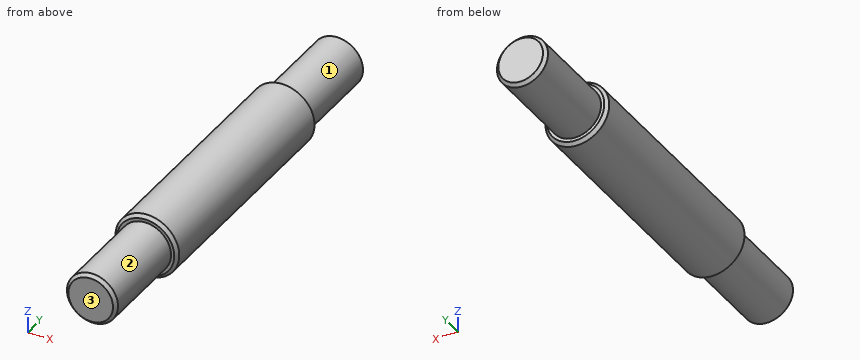
```python
from build123d import *

# Parameters (mm, degrees)
SKETCH1_R           = 5
BOSS_EXTRUDE1_DEPTH = 19
SKETCH2_R           = 4
BOSS_EXTRUDE2_DEPTH = 15
BOSS_EXTRUDE3_START = -53
SKETCH2_2_R         = 4
BOSS_EXTRUDE3_DEPTH = 15
CHAMFER1_SIZE       = 0.5
CHAMFER2_SIZE       = 0.5


with BuildPart() as part:
    # Sketch1 → Boss-Extrude1 (new, symmetric)
    with BuildSketch(Plane(origin=(0, 0, 0), x_dir=(1, 0, 0), z_dir=(0, 1, 0))):
        with Locations(Location((0, 0, 0), (0, 0, 270))):
            Circle(SKETCH1_R)
    extrude(amount=BOSS_EXTRUDE1_DEPTH, both=True)

    # Sketch2 → Boss-Extrude2 (add)
    with BuildSketch(Plane(origin=(0, 19, 0), x_dir=(1, 0, 0), z_dir=(0, 1, 0))):
        with Locations(Location((0, 0, 0), (0, 0, 270))):
            Circle(SKETCH2_R)
    extrude(amount=BOSS_EXTRUDE2_DEPTH)

    # Sketch2<2> → Boss-Extrude3 (add)
    with BuildSketch(Plane(origin=(0, 19, 0), x_dir=(1, 0, 0), z_dir=(0, 1, 0)).offset(BOSS_EXTRUDE3_START)):
        with Locations(Location((0, 0, 0), (0, 0, 270))):
            Circle(SKETCH2_2_R)
    extrude(amount=BOSS_EXTRUDE3_DEPTH)

    # Chamfer1
    chamfer1_edges = [part.edges().sort_by_distance(p)[0] for p in [
        (0, -34, -4),
        (0, 34, -4),
    ]]
    chamfer(chamfer1_edges, length=CHAMFER1_SIZE)

    # Chamfer2
    chamfer2_edges = [part.edges().sort_by_distance(p)[0] for p in [
        (0, -19, -5),
        (0, 19, -5),
    ]]
    chamfer(chamfer2_edges, length=CHAMFER2_SIZE)


solid = part.part
```
Design review of the part built by this model. Coordinates are the model's own, in mm. Face numbers are marked on the shaded views. A direction names the side the tool comes from. Round coordinates to 2 decimals unless told otherwise and drop trailing zeros. Write each loop counter-clockwise with the first axis right and the second up, starting at its lowest first coordinate (ties: lowest second). Pieces come first, ordered by that corner, then holes.
Item 1: Clearance check with a flat-ended pin moving along its axis: pin 1 Ø2 at (y, z) = (15.5, -3) entering from +X. State where the tip first meets the part, or that it passes through.
Item 2: We need section A-A on z = 0. Write out the cut boundary in (x, y).
Item 3: We need section C-C on y = -6.5. Write out the cut boundary in (x, z), and give its area (3 significant figures).
Item 4: We need section B-B on x = 0. Write out the cut boundary in (y, z).
Item 5: We need section D-D on y = 22.5. Write out the cut boundary in (x, z), and give its area (3 significant figures).
Item 6: For the marked faces 1, 2 and 3, list the 3-axis set-ups (+Z, -Z, +X, -X, +Y, -Y) from which the entire face can be reached by the end or side of a thin tool; tool diameter is ignored.
Item 7: For probe 1 along X at (y, z) = (-28, -0.25); probe 2 along Y at (x, z) = (4, -1); probe 3 along Z at (x, y) = (0.25, 13.5), list the stretches that pass through material, from the lowest coordinate up.
Returned:
1. pin 1: stops at x = 4.58
2. outline: (-5, -18.5) - (-4.5, -19) - (-4, -19) - (-4, -33.5) - (-3.5, -34) - (3.5, -34) - (4, -33.5) - (4, -19) - (4.5, -19) - (5, -18.5) - (5, 18.5) - (4.5, 19) - (4, 19) - (4, 33.5) - (3.5, 34) - (-3.5, 34) - (-4, 33.5) - (-4, 19) - (-4.5, 19) - (-5, 18.5) - close
3. outline: circle Ø10 at (0, 0)
3. area: 78.5 mm2
4. outline: (-34, -3.5) - (-33.5, -4) - (-19, -4) - (-19, -4.5) - (-18.5, -5) - (18.5, -5) - (19, -4.5) - (19, -4) - (33.5, -4) - (34, -3.5) - (34, 3.5) - (33.5, 4) - (19, 4) - (19, 4.5) - (18.5, 5) - (-18.5, 5) - (-19, 4.5) - (-19, 4) - (-33.5, 4) - (-34, 3.5) - close
5. outline: circle Ø8 at (0, 0)
5. area: 50.3 mm2
6. face 1: +Y
6. face 2: -Y
6. face 3: +Z, -Z, +X, -X, -Y
7. probe 1: x = -3.99 to 3.99
7. probe 2: y = -19 to 19
7. probe 3: z = -4.99 to 4.99
